```python
from build123d import *

# Parameters (mm, degrees)
F0_W     = 46.8510227791
F0_H     = 10.859509725
F1_DEPTH = 68.326
F2_DEPTH = 25.4
F4_R     = 635
F5_DEPTH = 805.18


with BuildPart() as f1:
    # F0 (on Front) → F1 (new body)
    with BuildSketch(Plane.XZ):
        with BuildLine():
            Line((0, 19.9349565315), (0, 0))
            Line((0, 0), (35.5261108433, 0))
            Line((35.5261108433, 0), (35.5261108433, 2.7486670447))
            ThreePointArc((35.5261108433, 2.7486670447), (31.9945535762, 7.7510571327), (35.5261108433, 12.7534472207))
            Line((35.5261108433, 12.7534472207), (35.5261108433, 13.7660977894))
            ThreePointArc((35.5261108433, 13.7660977894), (34.1369679811, 16.9197345446), (32.468561842, 19.9349565315))
            Line((32.468561842, 19.9349565315), (0, 19.9349565315))
        make_face()
        with Locations((-6.2054333332, -14.9706080555)):
            Rectangle(F0_W, F0_H)
        Polygon((35.5261108433, 0), (0, 0), (0, 19.9349565315), (-29.6309447227, -9.540853193), (17.2200780563, -9.540853193), align=None)
    extrude(amount=F1_DEPTH)

    # F0 (on Front) → F2 (join)
    with BuildSketch(Plane.XZ):
        with BuildLine():
            Line((0, 19.9349565315), (0, 0))
            Line((0, 0), (35.5261108433, 0))
            Line((35.5261108433, 0), (35.5261108433, 2.7486670447))
            ThreePointArc((35.5261108433, 2.7486670447), (31.9945535762, 7.7510571327), (35.5261108433, 12.7534472207))
            Line((35.5261108433, 12.7534472207), (35.5261108433, 13.7660977894))
            ThreePointArc((35.5261108433, 13.7660977894), (34.1369679811, 16.9197345446), (32.468561842, 19.9349565315))
            Line((32.468561842, 19.9349565315), (0, 19.9349565315))
        make_face()
        with BuildLine():
            Line((35.5261108433, 2.7486670447), (35.5261108433, 0))
            Line((35.5261108433, 0), (17.2200780563, -9.540853193))
            Line((17.2200780563, -9.540853193), (17.2200780563, -20.400362918))
            Line((17.2200780563, -20.400362918), (-29.6309447227, -20.400362918))
            Line((-29.6309447227, -20.400362918), (-29.6309447227, -9.540853193))
            Line((-29.6309447227, -9.540853193), (0, 19.9349565315))
            Line((0, 19.9349565315), (32.468561842, 19.9349565315))
            ThreePointArc((32.468561842, 19.9349565315), (-36.6651210702, -10.3575526506), (38.1, 0))
            ThreePointArc((38.1, 0), (38.0796183926, 1.2460590178), (38.0184953766, 2.4907848763))
            ThreePointArc((38.0184953766, 2.4907848763), (36.7568701316, 2.4705690147), (35.5261108433, 2.7486670447))
        make_face()
        with BuildLine():
            Line((35.5261108433, 12.7534472207), (35.5261108433, 2.7486670447))
            ThreePointArc((35.5261108433, 2.7486670447), (36.7568701316, 2.4705690147), (38.0184953766, 2.4907848763))
            ThreePointArc((38.0184953766, 2.4907848763), (37.3032319421, 7.7510571327), (35.8637504709, 12.8608476456))
            ThreePointArc((35.8637504709, 12.8608476456), (35.6940343979, 12.8099650441), (35.5261108433, 12.7534472207))
        make_face()
        with BuildLine():
            Line((35.5261108433, 19.9349565315), (32.468561842, 19.9349565315))
            ThreePointArc((32.468561842, 19.9349565315), (34.1369679811, 16.9197345446), (35.5261108433, 13.7660977894))
            Line((35.5261108433, 13.7660977894), (35.5261108433, 19.9349565315))
        make_face()
        with BuildLine():
            Line((35.5261108433, 13.7660977894), (35.5261108433, 12.7534472207))
            ThreePointArc((35.5261108433, 12.7534472207), (35.6940343979, 12.8099650441), (35.8637504709, 12.8608476456))
            ThreePointArc((35.8637504709, 12.8608476456), (35.6978002694, 13.3145430237), (35.5261108433, 13.7660977894))
        make_face()
        with BuildLine():
            ThreePointArc((35.8637504709, 12.8608476456), (37.3032319421, 7.7510571327), (38.0184953766, 2.4907848763))
            ThreePointArc((38.0184953766, 2.4907848763), (41.3019298247, 4.2592837672), (42.611910308, 7.7510571327))
            ThreePointArc((42.611910308, 7.7510571327), (40.5079411214, 11.9833029984), (35.8637504709, 12.8608476456))
        make_face()
    extrude(amount=F2_DEPTH)


with BuildPart() as f5:
    # F4 (on Front) → F5 (new body)
    with BuildSketch(Plane.XZ):
        Circle(F4_R)
    extrude(amount=F5_DEPTH)


solid = f5.part
```
Work out the finished part from the listing and answer in its coordinate system (mm). Give positions to 0.01 mm unless a question says otherwise; leave off trailing zeros. Order: outer loops, then holes, each group sorted by start corner. A loop starts at its lowest first (then second) coordinate and runs counter-clockwise, first axis right, second up. Notation, with made-up numbers: M -35,50 L -12,50 A19 cw -12,73 Z; hole C -2.75,-29 d4. An arc over 180 degrees is marked long. Return JSON: item names as keys, results as strings.
1) Straight lines are drawn through the part: line 1 along X through (y, z) = (-359, 466.5); line 2 along X through (y, z) = (-227, -471); line 3 along Z through (x, y) = (502.5, -290). For each, find the intervals that lie inside material, in ascending order. Write a range as [from, to].
Resolved:
{"line 1": "[-430.82, 430.82]", "line 2": "[-425.89, 425.89]", "line 3": "[-388.23, 388.23]"}
2) Each of these flat-tipped pins is pushed along its axis until it touches: pin 1 (3 mm diameter, centred on x = -199, y = -603.5, fed in from +Z); pin 2 (5 mm diameter, centred on x = -387, y = -628, fed in from -Z); pin 3 (5 mm diameter, centred on x = 179.5, y = -721.5, fed in from -Z); pin 4 (1 mm diameter, centred on x = 497.5, z = -367, fed in from +Y). Where does it stop, or does it pass through?
Resolved:
{"pin 1": "z = 603.51", "pin 2": "z = -505.36", "pin 3": "z = -609.83", "pin 4": "y = 0"}
3) Section C-C, the plane x = -113.5 is taken. Write down the section's boundary in (y, z).
Resolved:
{"outline": "M -805.18,-624.77 L 0,-624.77 L 0,624.77 L -805.18,624.77 Z"}
4) Section B-B, the plane z = 513 is taken. Write down the section's boundary in (x, y), plus the area to 3 significant figures.
Resolved:
{"outline": "M -374.24,-805.18 L 374.24,-805.18 L 374.24,0 L -374.24,0 Z", "area": "603,000 mm^2"}
5) Section A-A, the plane y = -688.5 is taken. Write down the section's boundary in (x, z), plus the area to 3 significant figures.
Resolved:
{"outline": "C 0,0 d1270", "area": "1,270,000 mm^2"}
